Here's how the part is built. I have some questions about the finished solid (model axes, mm). Face numbers are marked on the shaded views. A direction names the side the tool comes from. Round coordinates to 2 decimals unless told otherwise and drop trailing zeros. Write each loop counter-clockwise with the first axis right and the second up, starting at its lowest first coordinate (ties: lowest second). Pieces come first, ordered by that corner, then holes. Notation, with made-up numbers: (-29.75, 87) -> (15.25, 87) arc R28 cw to (15.25, 126) -> close; hole circle Ø4 at (87, 85.5). An arc over 180 degrees is marked (long way). Put each result on its own line as item: value. Start each with the question number.
1. Suppose I cut it at C-C (z = 88). Please give me the cut outline in (x, y).
2. We'd pull the mould along Y, two halves only. Please class the marked faces 1, 2 and 3: +Y half, -Y half, draft (parallel to the pull), parting line (faces both ways), or undercut.
3. Which directions (+Z, -Z, +X, -X, +Y, -Y) give clear straight access to the entire face, cutting with the end or side of a thin tool? Please do the marked faces 4, 5, 6 and 7.
4. For pin 1 (2 mm diameter, centred on x = -2.5, z = 84.5, fed in from -Y); pin 2 (3 mm diameter, centred on x = -28, y = -3, fed in from +Z); pin 3 (15 mm diameter, centred on x = -8.5, z = 9.5, fed in from -Y); pin 4 (1.5 mm diameter, centred on y = 15.5, z = 37, fed in from -X), each with a flat end and sliding along its axis, tell me the tip position at first contact or that it passes through.
5. I need wall thicknesses on probe 1 along X at (y, z) = (14.15, 20); probe 2 along Y at (x, z) = (11, 24); probe 3 along Y at (x, z) = (-21.5, 0.5). Which ranges of each line are inside material? Lowest first, please. Write a range as from..to.
6. Suppose I cut it at B-B (z = 65.5). Please give me the cut outline in (x, y), then the cut area to 3 significant figures.
7. Suppose I cut it at A-A (z = 20). Please give me the cut outline in (x, y), then the cut area to 4 significant figures.
8. Suppose I cut it at D-D (y = -29.5). Please give me the cut outline in (x, z).
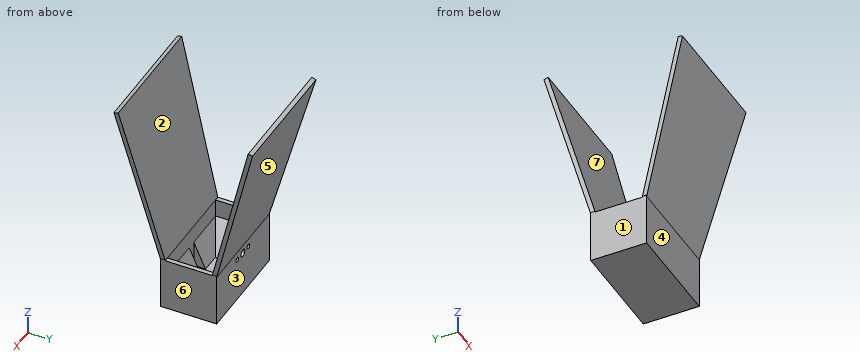
```python
from build123d import *

# Parameters (mm, degrees)
CROQUIS1_W                   = 53
CROQUIS1_H                   = 26.5
SALIENTE_EXTRUIR1_DEPTH      = 14.8
CROQUIS8_W                   = 5
CROQUIS8_H                   = 26.5
CORTAR_EXTRUIR2_DEPTH        = 14.8
SALIENTE_EXTRUIR2_DEPTH      = 35
SALIENTE_EXTRUIR2_DEPTH_BACK = 35
CROQUIS12_W                  = 2.5
CROQUIS12_H                  = 26.5
SALIENTE_EXTRUIR3_DEPTH      = 25
CORTAR_EXTRUIR3_DEPTH        = 31.5
CORTAR_EXTRUIR13_DEPTH       = 2.5
CORTAR_EXTRUIR14_DEPTH       = 2.5
CORTAR_EXTRUIR11_START       = -30.5
CORTAR_EXTRUIR11_OUTLINE_W   = 6
CORTAR_EXTRUIR11_OUTLINE_H   = 2.5
CORTAR_EXTRUIR11_DEPTH       = 0.819228498
CROQUIS18_R                  = 2.1
CROQUIS18_R_2                = 1.35
CORTAR_EXTRUIR12_DEPTH       = 2.5


# Read off the part's stored shape, not the designer's step: Cortar-Extruir11
with BuildPart() as part:
    # Croquis1 → Saliente-Extruir1 (new body)
    with BuildSketch(Plane.XY):
        Rectangle(CROQUIS1_W, CROQUIS1_H)
    extrude(amount=SALIENTE_EXTRUIR1_DEPTH)

    # Croquis5 → Cortar-Recubrir3 section 0
    with BuildSketch(Plane.XY.offset(14.8)):
        with BuildLine():
            Line((-26.5, 13.25), (-26.5, -13.25))
            Line((-26.5, -13.25), (26.5, -13.25))
            Line((26.5, -13.25), (26.5, 13.25))
            Line((26.5, 13.25), (-26.5, 13.25))
        make_face()
    # Croquis6 → Cortar-Recubrir3 section 1
    with BuildSketch(Plane(origin=(0, 0, 0), x_dir=(-1, 0, 0), z_dir=(0, 0, -1))):
        with BuildLine():
            Line((-13.25, -6.625), (13.25, -6.625))
            Line((13.25, -6.625), (13.25, 6.625))
            Line((13.25, 6.625), (-13.25, 6.625))
            Line((-13.25, 6.625), (-13.25, -6.625))
        make_face()
    loft(mode=Mode.SUBTRACT)

    # Croquis8 → Cortar-Extruir2 (cut)
    with BuildSketch(Plane(origin=(0, 0, 0), x_dir=(-1, 0, 0), z_dir=(0, 0, -1))):
        Rectangle(CROQUIS8_W, CROQUIS8_H)
    extrude(amount=-CORTAR_EXTRUIR2_DEPTH, mode=Mode.SUBTRACT)


with BuildPart() as cortar_extruir2_piece_1:
    # of the separate pieces the step leaves, piece 1, a body of its own (cortar_extruir2_pieces)
    add(part.part.solids().sort_by_distance((-26.5, -13.25, 0))[0])



with BuildPart() as cortar_extruir2_piece_2:
    # of the separate pieces the step leaves, piece 2, a body of its own (cortar_extruir2_pieces)
    add(part.part.solids().sort_by_distance((2.5, -13.25, 0))[0])


with BuildPart() as cortar_extruir2_piece_1_1:
    add(cortar_extruir2_piece_1.part)

    add(cortar_extruir2_piece_2.part)  # Saliente-Extruir2 merges Cortar-Extruir2 piece 2
    # Croquis10 → Saliente-Extruir2 (add, two sides: drawn at the far end of the back side and taken through both)
    with BuildSketch(Plane(origin=(0, 0, 0), x_dir=(0, 0, -1), z_dir=(1, 0, 0)).offset(-SALIENTE_EXTRUIR2_DEPTH_BACK)):
        Polygon((-14.8, 13.25), (-25, 13.25), (-115, 36.615427319), (-114.371786091, 39.035209806), (-24.680771502, 15.75), (5, 15.75), (5, 15), (5, -15.75), (-24.680771502, -15.75), (-114.371786091, -39.035209806), (-115, -36.615427319), (-25, -13.25), (-14.8, -13.25), (0, -13.25), (0, 13.25), align=None)
    extrude(amount=SALIENTE_EXTRUIR2_DEPTH + SALIENTE_EXTRUIR2_DEPTH_BACK)

    # Croquis12 → Saliente-Extruir3 (add)
    with BuildSketch(Plane.XY):
        with Locations((-27.75, 0)):
            Rectangle(CROQUIS12_W, CROQUIS12_H)
        with Locations((27.75, 0)):
            Rectangle(CROQUIS12_W, CROQUIS12_H)
    extrude(amount=SALIENTE_EXTRUIR3_DEPTH)

    # Croquis13 → Cortar-Extruir3 (cut)
    with BuildSketch(Plane(origin=(0, 15.75, 0), x_dir=(1, 0, 0), z_dir=(0, 1, 0))):
        Polygon((-35, 5), (-35, -24.680771502), (-29, -22.136705373), (-29, 2.455933871), align=None)
        Polygon((-29, 5), (-35, 5), (-29, 2.455933871), align=None)
        Polygon((-29, -22.136705373), (-35, -24.680771502), (-29, -24.680771502), align=None)
        Polygon((29, -22.136705373), (29, -24.680771502), (35, -24.680771502), align=None)
        Polygon((35, 5), (29, 2.455933871), (29, -22.136705373), (35, -24.680771502), align=None)
        Polygon((29, 5), (29, 2.455933871), (35, 5), align=None)
    extrude(amount=-CORTAR_EXTRUIR3_DEPTH, mode=Mode.SUBTRACT)

    # Croquis14 → Cortar-Extruir13 (cut)
    with BuildSketch(Plane(origin=(0, 8.752554668, -2.272301999), x_dir=(1, 0, 0), z_dir=(0, 0.9679129947926777, -0.25128556367501503))):
        Polygon((29, -27.846587086), (35, -27.846587086), (35, -120.510922694), align=None)
        Polygon((-35, -120.510922694), (-35, -27.846587086), (-29, -27.846587086), align=None)
    extrude(amount=-CORTAR_EXTRUIR13_DEPTH, mode=Mode.SUBTRACT)

    # Croquis16 → Cortar-Extruir14 (cut)
    with BuildSketch(Plane(origin=(0, -8.752554668, -2.272301999), x_dir=(1, 0, 0), z_dir=(0, -0.9679129947926624, -0.25128556367507404))):
        Polygon((-29, 27.846587086), (-35, 27.846587086), (-35, 120.510922694), align=None)
        Polygon((35, 120.510922694), (35, 27.846587086), (29, 27.846587086), align=None)
    extrude(amount=-CORTAR_EXTRUIR14_DEPTH, mode=Mode.SUBTRACT)

    # Cortar-Extruir11 outline → Cortar-Extruir11 (cut)
    with BuildSketch(Plane(origin=(0, 0, -5), x_dir=(-1, 0, 0), z_dir=(0, 0, -1)).offset(CORTAR_EXTRUIR11_START)):
        with Locations((-32, -14.5)):
            Rectangle(CORTAR_EXTRUIR11_OUTLINE_W, CORTAR_EXTRUIR11_OUTLINE_H)
        with Locations((32, -14.5)):
            Rectangle(CORTAR_EXTRUIR11_OUTLINE_W, CORTAR_EXTRUIR11_OUTLINE_H)
        with Locations((-32, 14.5)):
            Rectangle(CORTAR_EXTRUIR11_OUTLINE_W, CORTAR_EXTRUIR11_OUTLINE_H)
        with Locations((32, 14.5)):
            Rectangle(CORTAR_EXTRUIR11_OUTLINE_W, CORTAR_EXTRUIR11_OUTLINE_H)
    extrude(amount=CORTAR_EXTRUIR11_DEPTH, mode=Mode.SUBTRACT)

    # Croquis18 → Cortar-Extruir12 (cut)
    with BuildSketch(Plane(origin=(0, 15.75, 0), x_dir=(1, 0, 0), z_dir=(0, 1, 0))):
        with Locations(Location((0.081355667, -19.999867625, 0), (0, 0, 270))):
            Circle(CROQUIS18_R)
        with Locations(Location((6.181355666, -20, 0), (0, 0, 270))):
            Circle(CROQUIS18_R_2)
        with Locations(Location((-6.018644331, -20, 0), (0, 0, 270))):
            Circle(CROQUIS18_R_2)
    extrude(amount=-CORTAR_EXTRUIR12_DEPTH, mode=Mode.SUBTRACT)


solid = cortar_extruir2_piece_1_1.part
```
Verdict:
1. outline: (-33.24, -32.19) -> (33.24, -32.19) -> (33.19, -29.61) -> (-33.19, -29.61) -> close; (-33.24, 32.19) -> (-33.19, 29.61) -> (33.19, 29.61) -> (33.24, 32.19) -> close
2. face 1: draft
2. face 2: undercut
2. face 3: +Y half
3. face 4: -Z, +X, -X, -Y
3. face 5: -Z, +X, -X, +Y
3. face 6: -Z, +X, +Y, -Y
3. face 7: +Z, +X, -X
4. pin 1: stops at y = -31.54
4. pin 2: stops at z = 25
4. pin 3: stops at y = -15.75
4. pin 4: passes through
5. probe 1: x = -29..-7.37, -4.67..-2.02, 2.18..4.83, 7.53..29
5. probe 2: y = -15.75..-13.25, 13.25..15.75
5. probe 3: y = -15.75..15.75
6. outline: (-31.73, -26.35) -> (31.73, -26.35) -> (31.69, -23.76) -> (-31.69, -23.76) -> close; (-31.73, 26.35) -> (-31.69, 23.76) -> (31.69, 23.76) -> (31.73, 26.35) -> close
6. area: 328 mm^2
7. outline: (-29, -15.75) -> (29, -15.75) -> (29, 15.75) -> (7.53, 15.75) -> (7.53, 13.25) -> (26.5, 13.25) -> (26.5, -13.25) -> (-26.5, -13.25) -> (-26.5, 13.25) -> (-7.37, 13.25) -> (-7.37, 15.75) -> (-29, 15.75) -> close; (-4.67, 13.25) -> (-2.02, 13.25) -> (-2.02, 15.75) -> (-4.67, 15.75) -> close; (2.18, 13.25) -> (4.83, 13.25) -> (4.83, 15.75) -> (2.18, 15.75) -> close
7. area: 398.5 mm^2
8. outline: (-33.17, 87.59) -> (-32.54, 77.64) -> (32.54, 77.64) -> (33.17, 87.59) -> close
